The listing builds one solid part. Answer for the finished solid, in the listing's coordinates (mm). Face numbers are marked on the shaded views. A direction names the side the tool comes from. Coordinates: 2 decimals unless noted, no trailing zeros. Order: outer loops, then holes, each group sorted by start corner. A loop starts at its lowest first (then second) coordinate and runs counter-clockwise, first axis right, second up.
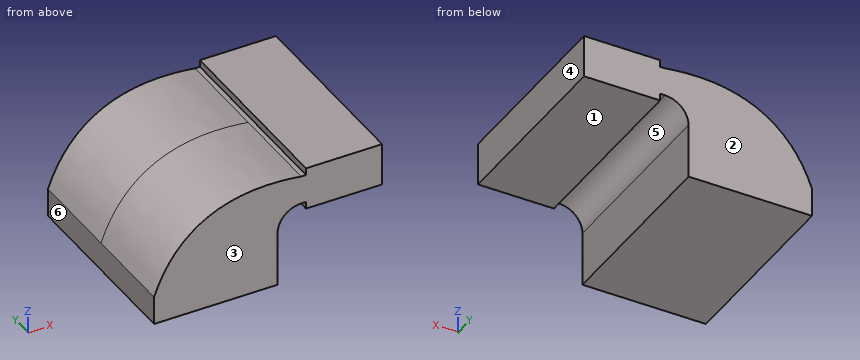
```python
from build123d import *

# Parameters (mm, degrees)
F0_W     = 20.1580673288
F0_H     = 19.05
F1_DEPTH = 63.5


with BuildPart() as f1:
    # F0 (on Front) → F1 (new body, symmetric)
    with BuildSketch(Plane.XZ):
        with BuildLine():
            Line((22.225, 9.525), (41.275, 9.525))
            Line((41.275, 9.525), (41.275, 27.0002))
            ThreePointArc((41.275, 27.0002), (45.9246798487, 38.2255201513), (57.15, 42.8752))
            Line((57.15, 42.8752), (60.325, 42.8752))
            Line((60.325, 42.8752), (60.325, 61.9252))
            Line((60.325, 61.9252), (57.15, 61.9252))
            ThreePointArc((57.15, 61.9252), (32.4542956671, 51.6959043329), (22.225, 27.0002))
            Line((22.225, 27.0002), (22.225, 9.525))
        make_face()
        with BuildLine():
            add(Edge.make_bspline(
                [(-41.275, 9.525), (-24.4504585862, 56.9105558097), (13.9114698395, 68.2926625013), (57.15, 61.9252)],
                knots=[0, 0, 0, 0, 111.5045361635, 111.5045361635, 111.5045361635, 111.5045361635], degree=3))
            Line((-41.275, 9.525), (22.225, 9.525))
            Line((22.225, 9.525), (22.225, 27.0002))
            ThreePointArc((22.225, 27.0002), (32.4542956671, 51.6959043329), (57.15, 61.9252))
        make_face()
        with Locations((70.4040336644, 52.4002)):
            Rectangle(F0_W, F0_H)
        Polygon((60.325, 66.675), (60.325, 61.9252), (80.4830673288, 61.9252), (80.4830673288, 42.8752), (60.325, 42.8752), (60.325, 38.1), (111.125, 38.1), (111.125, 66.675), align=None)
        Polygon((-41.275, 9.525), (-41.275, -9.525), (41.275, -9.525), (41.275, 9.525), (22.225, 9.525), align=None)
    extrude(amount=F1_DEPTH, both=True)


solid = f1.part
```
(1) Each of these flat-tipped pins is pushed along its axis until it touches: pin 1 Ø1.6 at (x, y) = (58.5, -25) entering from +Z; pin 2 Ø4 at (y, z) = (15.5, 2.5) entering from +X (3 decimals); pin 3 Ø3.5 at (x, y) = (59, -8.5) entering from -Z. Where does it stop, or does it pass through?
(2) For the marked faces 1 and 2, determine the directions among +Z, -Z, +X, -X, +Y, -Y from which every point of the face is accessible in a straight line to the end or side of a thin tool.
(3) Find section A-A (x = 76). Write down the section's boundary in (y, z) (3 decimals).
(4) The mould has two halves that part along X. Classify the marked faces 3, 4, 5 and 6: released by +X, released by -X, zero draft, split by the parting line, or undercut.
(5) Find section B-B (z = 2.5). Write down the section's boundary in (x, y) (3 decimals), and give its area (3 significant figures).
(6) Consider line 1 (Z direction, x = 90.5, y = -12) (3 decimals); line 2 (X direction, y = -37.5, z = 4.5) (3 decimals); line 3 (X direction, y = -57, z = 39) (3 decimals). Determine where each line is inside the solid, lowest interval first.
Findings below:
1. pin 1: stops at z = 61.93
1. pin 2: stops at x = 41.275
1. pin 3: stops at z = 38.1
2. face 1: -Z, +X, +Y, -Y
2. face 2: +Z, -Z, +X, -X, +Y
3. outline: (-63.5, 38.1) - (63.5, 38.1) - (63.5, 66.675) - (-63.5, 66.675) - close
4. face 3: zero draft
4. face 4: released by +X
4. face 5: undercut
4. face 6: released by -X
5. outline: (-41.275, -63.5) - (41.275, -63.5) - (41.275, 63.5) - (-41.275, 63.5) - close
5. area: 10,500 mm2
6. line 1: z = 38.1 to 66.675
6. line 2: x = -41.275 to 41.275
6. line 3: x = -24.527 to 46.757, 60.325 to 111.125
